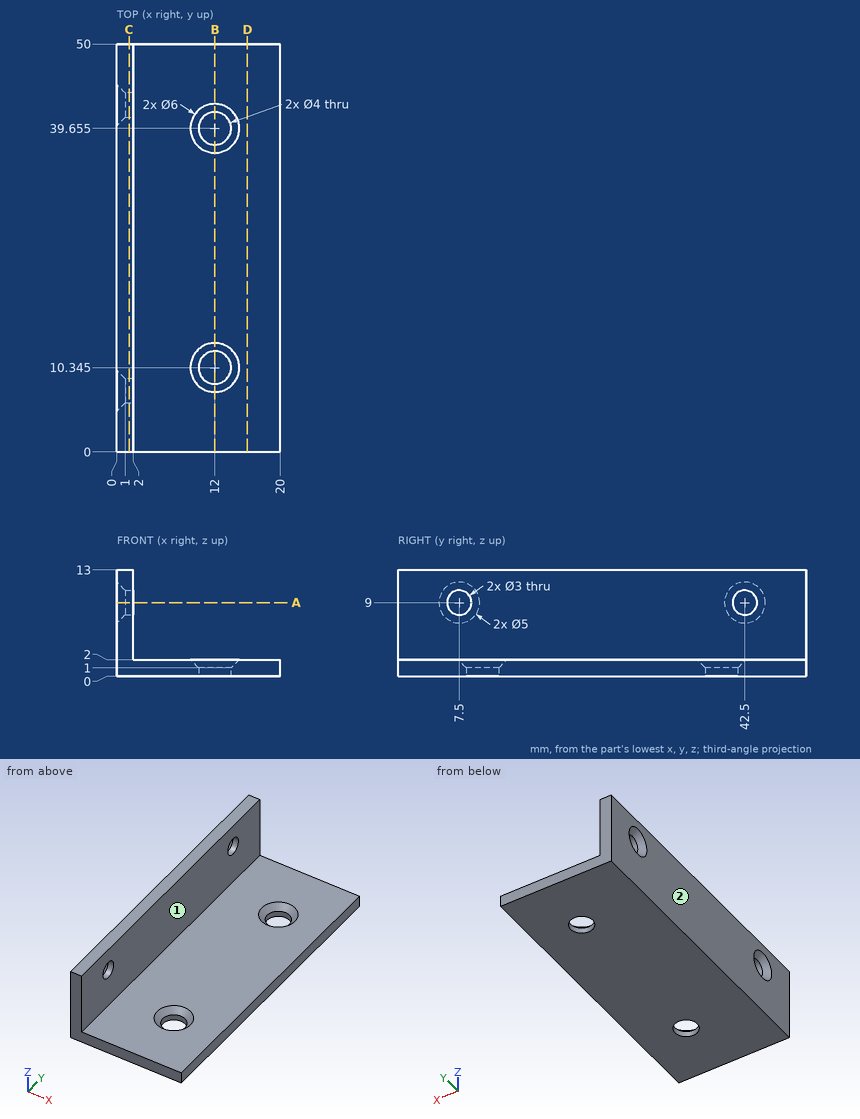
Geometry check sheet. Reference: drawing and pictorial views, mm from the part's lowest x, y, z. A direction names the side the tool comes from. Round coordinates to 2 decimals unless told otherwise and drop trailing zeros. Loops run counter-clockwise (first coordinate to the right, second up) from the corner with the lowest first, then second, coordinate; pieces in that order, holes last. Notation, with made-up numbers: (81, 37) -> (89, 37) arc R25 ccw to (89, 52) -> close; hole circle Ø6 at (69, 80.5). An arc over 180 degrees is marked (long way). Answer as a JSON object with one key per item and string values. Group by question number.
Item 1: Set-up check for the marked faces 1 and 2: record each of +Z, -Z, +X, -X, +Y, -Y from which the full face is reachable in a straight line by a thin tool's end or side.
Item 2: Cross-section at B-B, the plane x = 12. Record the cut outline in (y, z) (3 decimals).
Item 3: Thickness scan on line 1 along Y through (x, z) = (12, 0.3) (3 decimals); line 2 along Z through (x, y) = (9.25, 13). Record the ranges inside material, lowest first.
Item 4: Depth check by flat-ended pin: pin 1 Ø5.5 at (y, z) = (34.5, 9.5) entering from +X; pin 2 Ø5.5 at (x, y) = (13, 22.5) entering from +Z. Enter the tip coordinate at first touch or a pass-through.
Item 5: Cross-section at D-D, the plane x = 16. Record the cut outline in (y, z).
Item 6: Cross-section at A-A, the plane z = 9. Record the cut outline in (x, y).
Item 7: Cross-section at C-C, the plane x = 1.5. Record the cut outline in (y, z).
Determined:
{
 "1": {"face 1": "+Z, +X, +Y, -Y", "face 2": "+Z, -Z, -X, +Y, -Y"},
 "2": {"outline": "(0, 0) -> (8.345, 0) -> (8.345, 1) -> (7.345, 2) -> (0, 2) -> close; (12.345, 0) -> (37.655, 0) -> (37.655, 1) -> (36.655, 2) -> (13.345, 2) -> (12.345, 1) -> close; (41.655, 0) -> (50, 0) -> (50, 2) -> (42.655, 2) -> (41.655, 1) -> close"},
 "3": {"line 1": "y = 0 to 8.345, 12.345 to 37.655, 41.655 to 50", "line 2": "z = 0 to 2"},
 "4": {"pin 1": "stops at x = 2", "pin 2": "stops at z = 2"},
 "5": {"outline": "(0, 0) -> (50, 0) -> (50, 2) -> (0, 2) -> close"},
 "6": {"outline": "(0, 0) -> (2, 0) -> (2, 6) -> (1, 6) -> (0, 5) -> close; (0, 10) -> (1, 9) -> (2, 9) -> (2, 41) -> (1, 41) -> (0, 40) -> close; (0, 45) -> (1, 44) -> (2, 44) -> (2, 50) -> (0, 50) -> close"},
 "7": {"outline": "(0, 0) -> (50, 0) -> (50, 13) -> (0, 13) -> close; hole circle Ø3 at (7.5, 9); hole circle Ø3 at (42.5, 9)"}
}
